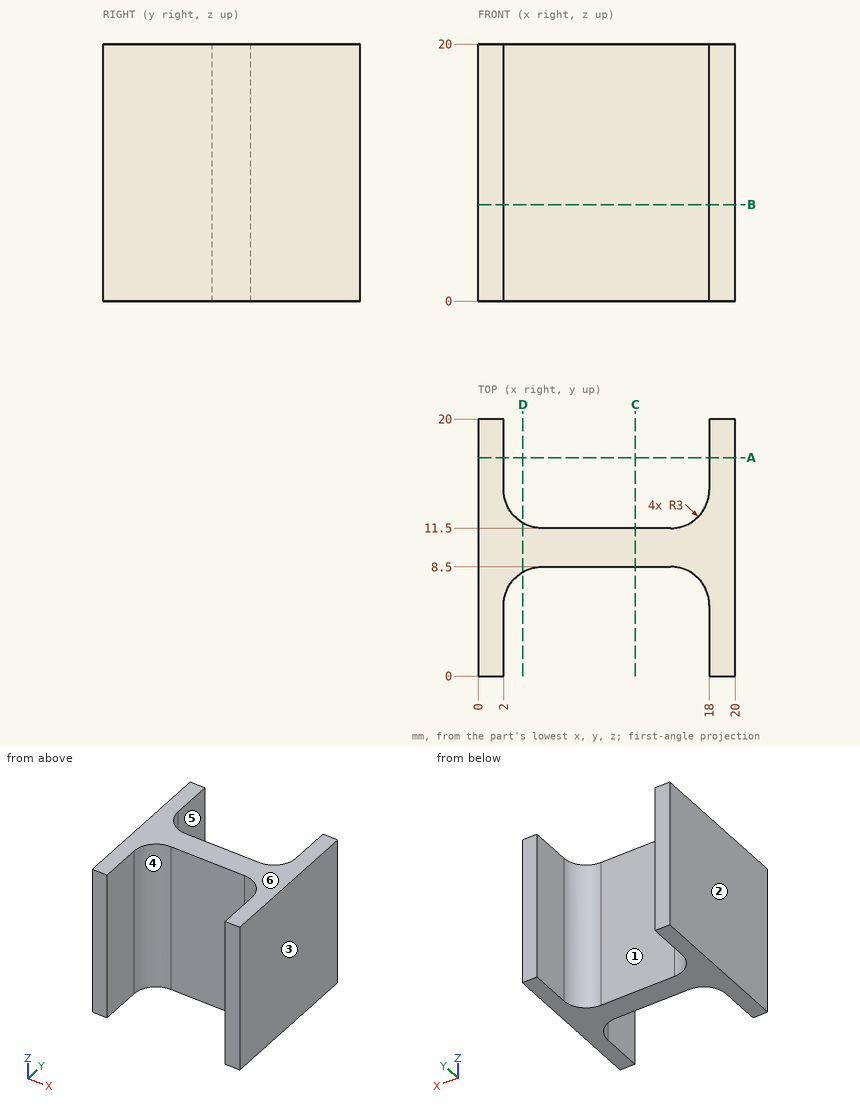
Could you check a few things on this drawing? It's one solid part, dimensions in mm from its lowest x, y, z. A direction names the side the tool comes from. Coordinates: 2 decimals unless noted, no trailing zeros. Write each loop counter-clockwise with the first axis right and the second up, starting at its lowest first coordinate (ties: lowest second). Pieces come first, ordered by that corner, then holes. Notation, with made-up numbers: M 53.5,72 L 57.5,72 A15 cw 57.5,96 Z; hole C 42.5,-30.75 d5. An arc over 180 degrees is marked long. Answer as CSV lines item,"result". Start each with the question number.
Q1. Suppose I cut it at C-C, the plane x = 12.25. List the corners of the cut face in (y, z) for me.
Q2. I need wall thicknesses on probe 1 along X at (y, z) = (2.25, 13); probe 2 along Y at (x, z) = (6, 4); probe 3 along X at (y, z) = (12, 12). Which ranges of each line are inside material? Lowest first, please. Write a range as [from, to].
Q3. Suppose I cut it at A-A, the plane y = 17. List the corners of the cut face in (x, z) for me.
Q4. Will these pins go through, and if not, where does the flat tip stop? pin 1 Ø3 at (x, z) = (8, 12) entering from +Y; pin 2 Ø5 at (x, z) = (11.5, 12.5) entering from -Y; pin 3 Ø12 at (x, z) = (11, 3) entering from -Y.
Q5. Suppose I cut it at B-B, the plane z = 7.5. List the corners of the cut face in (x, y) for me.
Q6. If we mould it in two halves opening along X, with no side actions, what happens to the marked faces 1, 2 and 3? For each: pulls with the +X half, pulls with the -X half, needs draft (parallel to the pull), parting line crosses it, or undercut.
Q7. For the marked faces 4, 5 and 6, which set-ups out of +Z, -Z, +X, -X, +Y, -Y let a thin tool reach every point of the face, with its end or its side?
Q8. Suppose I cut it at D-D, the plane x = 3.5. List the corners of the cut face in (y, z) for me, then the cut area to 3 significant figures.
Entries:
1,outline,"M 8.5,0 L 11.5,0 L 11.5,20 L 8.5,20 Z"
2,probe 1,"x = [0, 2], [18, 20]"
2,probe 2,"y = [8.5, 11.5]"
2,probe 3,"x = [0, 3.34], [16.66, 20]"
3,outline,"M 0,0 L 2,0 L 2,20 L 0,20 Z; M 18,0 L 20,0 L 20,20 L 18,20 Z"
4,pin 1,"stops at y = 11.5"
4,pin 2,"stops at y = 8.5"
4,pin 3,"stops at y = 7.74"
5,outline,"M 0,0 L 2,0 L 2,5.5 A3 cw 5,8.5 L 15,8.5 A3 cw 18,5.5 L 18,0 L 20,0 L 20,20 L 18,20 L 18,14.5 A3 cw 15,11.5 L 5,11.5 A3 cw 2,14.5 L 2,20 L 0,20 Z"
6,face 1,"undercut"
6,face 2,"pulls with the -X half"
6,face 3,"pulls with the +X half"
7,face 4,"+Z, -Z, -Y"
7,face 5,"+Z, -Z, +Y"
7,face 6,"+Z, +X, -X, +Y, -Y"
8,outline,"M 8.1,0 L 11.9,0 L 11.9,20 L 8.1,20 Z"
8,area,"76.1 mm²"
